```python
from build123d import *

# Parameters (mm, degrees)
BOSS_EXTRUDE1_DEPTH = 9.525
SKETCH3_W           = 28.575
SKETCH3_H           = 22.86
BOSS_EXTRUDE2_DEPTH = 50.8
FILLET1_R           = 5.08
SKETCH4_W           = 6.35
SKETCH4_H           = 22.225
SKETCH4_W_2         = 11.049
CUT_EXTRUDE1_DEPTH  = 143.837889922
FILLET3_R           = 11.43
SKETCH5_R           = 6.604
CUT_EXTRUDE2_DEPTH  = 172.690359797
SKETCH7_R           = 4.233333333
CUT_EXTRUDE3_DEPTH  = 5.08
SKETCH8_R           = 2.38125
CUT_EXTRUDE4_DEPTH  = 167.248859845
FILLET7_R           = 2.54


# Some blends are built 0.0001 mm under size
with BuildPart() as part:
    # Sketch1 → Boss-Extrude1 (new body)
    with BuildSketch(Plane.XY):
        Polygon((-11.895004803, 65.589219752), (11.895004803, 65.589219752), (60.958729286, 139.723968283), (76.844746829, 129.210313037), (14.2875, 34.687000521), (14.2875, -66.912999479), (-14.2875, -66.912999479), (-14.2875, 34.687000521), (-76.844746829, 129.210313037), (-60.958729286, 139.723968283), align=None)
    extrude(amount=BOSS_EXTRUDE1_DEPTH)

    # Sketch3 → Boss-Extrude2 (add)
    with BuildSketch(Plane.XY.offset(9.525)):
        with Locations((0, 50.138110136)):
            Rectangle(SKETCH3_W, SKETCH3_H)
    extrude(amount=BOSS_EXTRUDE2_DEPTH)

    # Fillet1
    fillet1_edges = [part.edges().sort_by_distance(p)[0] for p in [
        (-11.895004803, 65.589219752, 4.7625),
        (11.895004803, 65.589219752, 4.7625),
        (60.958729286, 139.723968283, 4.7625),
        (76.844746829, 129.210313037, 4.7625),
        (14.2875, 34.687000521, 4.7625),
        (14.2875, -66.912999479, 4.7625),
        (-14.2875, -66.912999479, 4.7625),
        (-14.2875, 34.687000521, 4.7625),
        (-76.844746829, 129.210313037, 4.7625),
        (-60.958729286, 139.723968283, 4.7625),
    ]]
    fillet(fillet1_edges, radius=FILLET1_R)

    # Sketch4 → Cut-Extrude1 (cut, through all)
    with BuildSketch(Plane.XZ.offset(-38.708110136)):
        with Locations((-11.1125, 49.2125)):
            Rectangle(SKETCH4_W, SKETCH4_H)
        with Locations((3.175, 49.2125)):
            Rectangle(SKETCH4_W_2, SKETCH4_H)
    extrude(amount=-CUT_EXTRUDE1_DEPTH, mode=Mode.SUBTRACT)

    # Fillet3
    fillet3_edges = [part.edges().sort_by_distance(p)[0] for p in [
        (11.4935, 61.568110136, 60.325),
        (-5.1435, 61.568110136, 60.325),
        (11.4935, 38.708110136, 60.325),
        (-5.1435, 38.708110136, 60.325),
    ]]
    fillet(fillet3_edges, radius=FILLET3_R - 0.0001)  # a hair under: the kernel refuses the full size

    # Sketch5 → Cut-Extrude2 (cut, through all)
    with BuildSketch(Plane.ZY.offset(7.9375)):
        with Locations(Location((48.895, 50.138110136, 0), (0, 0, 270))):
            Circle(SKETCH5_R)
    extrude(amount=-CUT_EXTRUDE2_DEPTH, mode=Mode.SUBTRACT)

    # Sketch7 → Cut-Extrude3 (cut)
    with BuildSketch(Plane(origin=(0, 0, 0), x_dir=(-1, 0, 0), z_dir=(0, 0, -1))):
        with Locations((0, -58.022999479)):
            Circle(SKETCH7_R)
    extrude(amount=-CUT_EXTRUDE3_DEPTH, mode=Mode.SUBTRACT)

    # Sketch8 → Cut-Extrude4 (cut, through all)
    with BuildSketch(Plane(origin=(0, 0, 5.08), x_dir=(-1, 0, 0), z_dir=(0, 0, -1))):
        with Locations((0, -58.022999479)):
            Circle(SKETCH8_R)
    extrude(amount=-CUT_EXTRUDE4_DEPTH, mode=Mode.SUBTRACT)

    # Fillet7
    # the kernel refuses this fillet: 2.54 mm, written as the material it adds along each edge
    with BuildSketch(Plane(origin=(-14.2875, 38.708110136, 9.525), x_dir=(0, 0, 1), z_dir=(0, 1, 0))) as fillet7_piece_1:
        with BuildLine():
            CenterArc((FILLET7_R, -FILLET7_R), FILLET7_R, 90, 90)
            Line((0, -FILLET7_R), (0, 0))
            Line((0, 0), (FILLET7_R, 0))
        make_face()
    extrude(amount=22.86)
    with BuildSketch(Plane(origin=(14.2875, 38.708110136, 9.525), x_dir=(0, 0, 1), z_dir=(-1, 0, 0))) as fillet7_piece_2:
        with BuildLine():
            CenterArc((FILLET7_R, -FILLET7_R), FILLET7_R, 90, 90)
            Line((0, -FILLET7_R), (0, 0))
            Line((0, 0), (FILLET7_R, 0))
        make_face()
    extrude(amount=28.575)
    with BuildSketch(Plane(origin=(14.2875, 61.568110136, 9.525), x_dir=(1, 0, 0), z_dir=(0, -1, 0))) as fillet7_piece_3:
        with BuildLine():
            CenterArc((FILLET7_R, FILLET7_R), FILLET7_R, 180, 90)
            Line((0, FILLET7_R), (0, 0))
            Line((0, 0), (FILLET7_R, 0))
        make_face()
    extrude(amount=22.86)
    with BuildSketch(Plane(origin=(-14.2875, 61.568110136, 9.525), x_dir=(0, 1, 0), z_dir=(1, 0, 0))) as fillet7_piece_4:
        with BuildLine():
            CenterArc((FILLET7_R, FILLET7_R), FILLET7_R, 180, 90)
            Line((0, FILLET7_R), (0, 0))
            Line((0, 0), (FILLET7_R, 0))
        make_face()
    extrude(amount=28.575)
    with BuildSketch(Plane(origin=(14.2875, 38.708110136, 9.525), x_dir=(0, 0, 1), z_dir=(-1, 0, 0))) as fillet7_piece_5a_section:
        with BuildLine():
            CenterArc((FILLET7_R, -FILLET7_R), FILLET7_R, 90, 90)
            Line((0, -FILLET7_R), (0, 0))
            Line((0, 0), (FILLET7_R, 0))
        make_face()
    fillet7_piece_5a = extrude(amount=34.925, mode=Mode.PRIVATE)
    fillet7_piece_5a = split(fillet7_piece_5a, bisect_by=Plane(origin=(-14.2875, 38.220078421, 10.151447049), z_dir=(-1, 0, 0)), keep=Keep.TOP, mode=Mode.PRIVATE)
    fillet7_piece_5a = split(fillet7_piece_5a, bisect_by=Plane(origin=(-16.26964909, 37.682006014, 10.151447049), z_dir=(0.8339116820223069, 0.5518979131929445, 0)), keep=Keep.TOP, mode=Mode.PRIVATE)
    with BuildSketch(Plane(origin=(-14.2875, 32.358110136, 9.525), x_dir=(0, 0, 1), z_dir=(0, 1, 0))) as fillet7_piece_5b_section:
        with BuildLine():
            CenterArc((FILLET7_R, -FILLET7_R), FILLET7_R, 90, 90)
            Line((0, -FILLET7_R), (0, 0))
            Line((0, 0), (FILLET7_R, 0))
        make_face()
    fillet7_piece_5b = extrude(amount=29.21, mode=Mode.PRIVATE)
    fillet7_piece_5b = split(fillet7_piece_5b, bisect_by=Plane(origin=(-14.718813993, 38.708110136, 10.184953821), z_dir=(0, -1, 0)), keep=Keep.TOP, mode=Mode.PRIVATE)
    fillet7_piece_5b = split(fillet7_piece_5b, bisect_by=Plane(origin=(-15.49417016, 36.510265873, 10.184953821), z_dir=(0.8339116820223069, 0.5518979131929445, 0)), keep=Keep.TOP, mode=Mode.PRIVATE)
    fillet7_piece_5 = fillet7_piece_5a & fillet7_piece_5b
    add(fillet7_piece_5)
    with BuildSketch(Plane(origin=(-14.2875, 38.708110136, 9.525), x_dir=(0, 0, 1), z_dir=(0, 1, 0))) as fillet7_piece_6a_section:
        with BuildLine():
            CenterArc((FILLET7_R, -FILLET7_R), FILLET7_R, 90, 90)
            Line((0, -FILLET7_R), (0, 0))
            Line((0, 0), (FILLET7_R, 0))
        make_face()
    fillet7_piece_6a = extrude(amount=29.21, mode=Mode.PRIVATE)
    fillet7_piece_6a = split(fillet7_piece_6a, bisect_by=Plane(origin=(-14.86254359, 61.568110136, 10.10004359), z_dir=(0, 1, 0)), keep=Keep.TOP, mode=Mode.PRIVATE)
    with BuildSketch(Plane(origin=(-20.6375, 61.568110136, 9.525), x_dir=(0, 1, 0), z_dir=(1, 0, 0))) as fillet7_piece_6b_section:
        with BuildLine():
            CenterArc((FILLET7_R, FILLET7_R), FILLET7_R, 180, 90)
            Line((0, FILLET7_R), (0, 0))
            Line((0, 0), (FILLET7_R, 0))
        make_face()
    fillet7_piece_6b = extrude(amount=34.925, mode=Mode.PRIVATE)
    fillet7_piece_6b = split(fillet7_piece_6b, bisect_by=Plane(origin=(-14.2875, 62.143153727, 10.10004359), z_dir=(-1, 0, 0)), keep=Keep.TOP, mode=Mode.PRIVATE)
    fillet7_piece_6 = fillet7_piece_6a & fillet7_piece_6b
    add(fillet7_piece_6)
    with BuildSketch(Plane(origin=(20.6375, 38.708110136, 9.525), x_dir=(0, 0, 1), z_dir=(-1, 0, 0))) as fillet7_piece_7a_section:
        with BuildLine():
            CenterArc((FILLET7_R, -FILLET7_R), FILLET7_R, 90, 90)
            Line((0, -FILLET7_R), (0, 0))
            Line((0, 0), (FILLET7_R, 0))
        make_face()
    fillet7_piece_7a = extrude(amount=34.925, mode=Mode.PRIVATE)
    fillet7_piece_7a = split(fillet7_piece_7a, bisect_by=Plane(origin=(14.2875, 38.220078421, 10.151447049), z_dir=(1, 0, 0)), keep=Keep.TOP, mode=Mode.PRIVATE)
    fillet7_piece_7a = split(fillet7_piece_7a, bisect_by=Plane(origin=(16.26964909, 37.682006014, 10.151447049), z_dir=(-0.8339116820223068, 0.5518979131929448, 0)), keep=Keep.TOP, mode=Mode.PRIVATE)
    with BuildSketch(Plane(origin=(14.2875, 61.568110136, 9.525), x_dir=(1, 0, 0), z_dir=(0, -1, 0))) as fillet7_piece_7b_section:
        with BuildLine():
            CenterArc((FILLET7_R, FILLET7_R), FILLET7_R, 180, 90)
            Line((0, FILLET7_R), (0, 0))
            Line((0, 0), (FILLET7_R, 0))
        make_face()
    fillet7_piece_7b = extrude(amount=29.21, mode=Mode.PRIVATE)
    fillet7_piece_7b = split(fillet7_piece_7b, bisect_by=Plane(origin=(14.718813993, 38.708110136, 10.184953821), z_dir=(0, -1, 0)), keep=Keep.TOP, mode=Mode.PRIVATE)
    fillet7_piece_7b = split(fillet7_piece_7b, bisect_by=Plane(origin=(15.49417016, 36.510265872, 10.184953821), z_dir=(-0.8339116820223068, 0.5518979131929448, 0)), keep=Keep.TOP, mode=Mode.PRIVATE)
    fillet7_piece_7 = fillet7_piece_7a & fillet7_piece_7b
    add(fillet7_piece_7)
    with BuildSketch(Plane(origin=(14.2875, 67.918110136, 9.525), x_dir=(1, 0, 0), z_dir=(0, -1, 0))) as fillet7_piece_8a_section:
        with BuildLine():
            CenterArc((FILLET7_R, FILLET7_R), FILLET7_R, 180, 90)
            Line((0, FILLET7_R), (0, 0))
            Line((0, 0), (FILLET7_R, 0))
        make_face()
    fillet7_piece_8a = extrude(amount=29.21, mode=Mode.PRIVATE)
    fillet7_piece_8a = split(fillet7_piece_8a, bisect_by=Plane(origin=(14.86254359, 61.568110136, 10.10004359), z_dir=(0, 1, 0)), keep=Keep.TOP, mode=Mode.PRIVATE)
    with BuildSketch(Plane(origin=(-14.2875, 61.568110136, 9.525), x_dir=(0, 1, 0), z_dir=(1, 0, 0))) as fillet7_piece_8b_section:
        with BuildLine():
            CenterArc((FILLET7_R, FILLET7_R), FILLET7_R, 180, 90)
            Line((0, FILLET7_R), (0, 0))
            Line((0, 0), (FILLET7_R, 0))
        make_face()
    fillet7_piece_8b = extrude(amount=34.925, mode=Mode.PRIVATE)
    fillet7_piece_8b = split(fillet7_piece_8b, bisect_by=Plane(origin=(14.2875, 62.143153727, 10.10004359), z_dir=(1, 0, 0)), keep=Keep.TOP, mode=Mode.PRIVATE)
    fillet7_piece_8 = fillet7_piece_8a & fillet7_piece_8b
    add(fillet7_piece_8)


solid = part.part
```
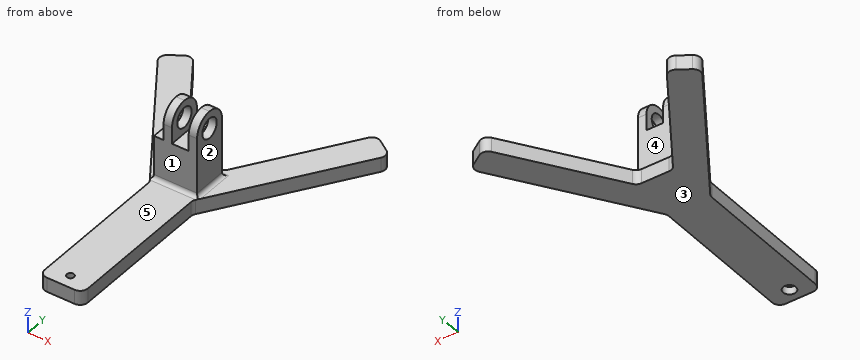
Geometry: final body of the model. Coordinates: model frame, mm. Face numbers are marked on the shaded views. A direction names the side the tool comes from. Coordinates: 2 decimals unless noted, no trailing zeros. Order: outer loops, then holes, each group sorted by start corner. A loop starts at its lowest first (then second) coordinate and runs counter-clockwise, first axis right, second up. Notation, with made-up numbers: M -6.75,-3 L -0.75,-3 A24 ccw -0.75,32 Z; hole C 68.25,31 d8. An arc over 180 degrees is marked long. Answer as CSV lines item,"result".
Q1. Section B-B on y = 110. Return the cut outline in (x, z) (3 decimals).
Answers:
outline,"M -64.131,0 L -41.287,0 L -41.287,9.525 L -64.131,9.525 Z; M 41.287,0 L 64.131,0 L 64.131,9.525 L 41.287,9.525 Z"
Q2. Section D-D on y = 20. Return the cut outline in (x, z) (1 decimal).
Answers:
outline,"M -14.3,0 L 14.3,0 L 14.3,9.5 L -14.3,9.5 Z"
Q3. Section C-C on z = 14.5. Return the cut outline in (x, y), and give its area (3 significant figures).
Answers:
outline,"M -14.29,38.71 L 14.29,38.71 L 14.29,61.57 L -14.29,61.57 Z"
area,"653 mm^2"
Q4. Line query: probe 1 along Y at (x, z) = (0, 1.3); probe 2 along X at (y, z) = (108.5, 5.5); probe 3 along X at (y, z) = (39.5, 29.5). Output: solid intervals per line, ascending. Write a range as [from, to].
Answers:
probe 1,"y = [-66.91, -62.26], [-53.79, 65.59]"
probe 2,"x = [-63.14, -40.29], [40.29, 63.14]"
probe 3,"x = [-14.29, 14.29]"
Q5. First-contact query: P1, Ø5.5, axis at x = 1.5, y = 55, coming from the +Z side; P2, Ø15.5, axis at x = -1, y = -9.5, coming from the +Z side (3 decimals); P3, Ø7.5, axis at x = 0, y = -58.023, coming from the -Z side; P4, Ø1.5, axis at x = -51.5, y = 108, coming from the -Z side. Flat tips, straight axial feed; report the tip coordinate or a pass-through.
Answers:
P1,"stops at z = 38.1"
P2,"stops at z = 9.525"
P3,"stops at z = 5.08"
P4,"stops at z = 0"
Q6. Set-up query: the marked faces 1 and 2. Return all of +Z, -Z, +X, -X, +Y, -Y with unobstructed straight access to the full face (end or side cutting, diameter ignored); none if empty.
Answers:
face 1,"+Z, +X, -X, -Y"
face 2,"+Z, +X, +Y, -Y"
Q7. Section A-A on x = 0. Return the cut outline in (y, z) (3 decimals).
Answers:
outline,"M -66.913,0 L -62.256,0 L -62.256,5.08 L -60.404,5.08 L -60.404,9.525 L -66.913,9.525 Z; M -55.642,5.08 L -53.79,5.08 L -53.79,0 L 65.589,0 L 65.589,9.525 L 64.108,9.525 A2.54 cw 61.568,12.065 L 61.568,38.1 L 38.708,38.1 L 38.708,12.065 A2.54 cw 36.168,9.525 L -55.642,9.525 Z"
Q8. Draft query along Z for the marked faces 3, 4 and 5. Return one class per face: pulls with the +Z half, pulls with the -Z half, needs draft (parallel to the pull), parting line crosses it, or undercut.
Answers:
face 3,"pulls with the -Z half"
face 4,"needs draft"
face 5,"pulls with the +Z half"
